Could you check a few things on this drawing? It's one solid part, dimensions in mm from its lowest x, y, z. Coordinates: 2 decimals unless noted, no trailing zeros. Write each loop counter-clockwise with the first axis right and the second up, starting at its lowest first coordinate (ties: lowest second). Pieces come first, ordered by that corner, then holes.
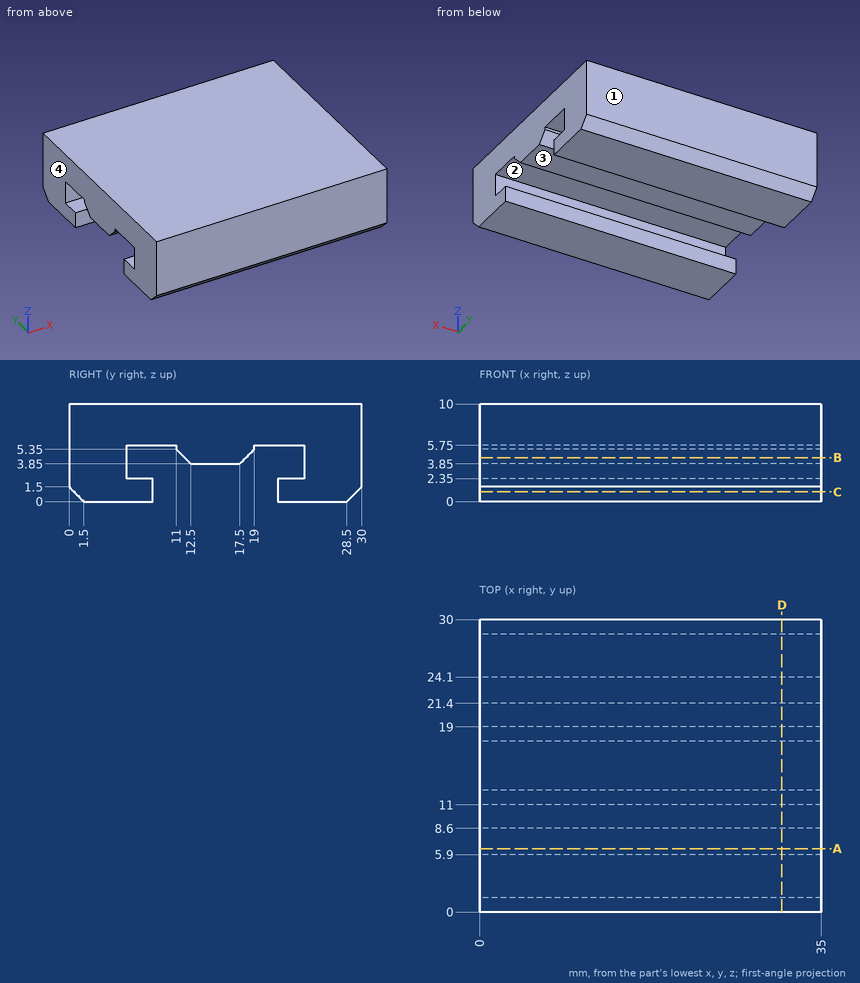
1) Imagine slicing it at A-A on y = 6.5. Please give me the cut outline in (x, z).
Values follow:
outline: (0, 0) - (35, 0) - (35, 2.35) - (0, 2.35) - close; (0, 5.75) - (35, 5.75) - (35, 10) - (0, 10) - close
2) Imagine slicing it at B-B on z = 4.5. Please give me the cut outline in (x, y), then the cut area to 4 significant figures.
Values follow:
outline: (0, 0) - (35, 0) - (35, 5.9) - (0, 5.9) - close; (0, 11.85) - (35, 11.85) - (35, 18.15) - (0, 18.15) - close; (0, 24.1) - (35, 24.1) - (35, 30) - (0, 30) - close
area: 633.5 mm2
3) Will these pins go through, and if not, where does the flat tip stop? pin 1 (3 mm diameter, centred on y = 10.5, z = 3, fed in from -X); pin 2 (1.2 mm diameter, centred on x = 13.5, z = 0.5, fed in from -Y); pin 3 (4 mm diameter, centred on x = 19.5, y = 14.5, fed in from -Z).
Values follow:
pin 1: passes through
pin 2: stops at y = 0.4
pin 3: stops at z = 3.85
4) We'd pull the mould along Y, two halves only. Please class the marked faces 1, 2, 3 and 4: pulls with the +Y half, pulls with the -Y half, needs draft (parallel to the pull), parting line crosses it, or undercut.
Values follow:
face 1: pulls with the +Y half
face 2: undercut
face 3: undercut
face 4: needs draft
5) I need wall thicknesses on probe 1 along Y at (x, z) = (16.5, 3.5); probe 2 along Z at (x, y) = (34, 22.5); probe 3 along Z at (x, y) = (5, 19.25). Which ranges of each line are inside material? Lowest first, please.
Values follow:
probe 1: y = 0 to 5.9, 24.1 to 30
probe 2: z = 0 to 2.35, 5.75 to 10
probe 3: z = 5.75 to 10
6) Imagine slicing it at D-D on x = 31. Please give me the cut outline in (y, z).
Values follow:
outline: (0, 1.5) - (1.5, 0) - (8.6, 0) - (8.6, 2.35) - (5.9, 2.35) - (5.9, 5.75) - (11, 5.75) - (11, 5.35) - (12.5, 3.85) - (17.5, 3.85) - (19, 5.35) - (19, 5.75) - (24.1, 5.75) - (24.1, 2.35) - (21.4, 2.35) - (21.4, 0) - (28.5, 0) - (30, 1.5) - (30, 10) - (0, 10) - close
7) Imagine slicing it at C-C on z = 1. Please give me the cut outline in (x, y).
Values follow:
outline: (0, 0.5) - (35, 0.5) - (35, 8.6) - (0, 8.6) - close; (0, 21.4) - (35, 21.4) - (35, 29.5) - (0, 29.5) - close
